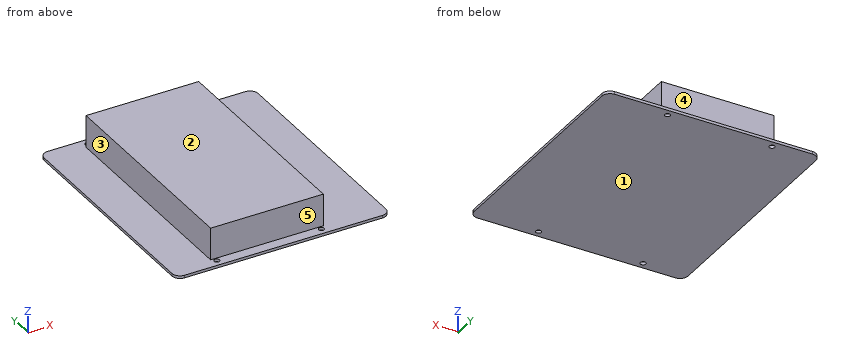
from build123d import *

# Parameters (mm, degrees)
BOSS_EXTRUDE1_DEPTH     = 1.27
SKETCH2_W               = 53.34
SKETCH2_H               = 101.981
BOSS_EXTRUDE2_DEPTH     = 15.24
CUT_EXTRUDE1_DEPTH      = 78.055045652
CUT_EXTRUDE1_DEPTH_BACK = 78.055045652
SKETCH4_R               = 1.27


with BuildPart() as part:
    # Sketch1 → Boss-Extrude1 (new body)
    with BuildSketch(Plane.XY):
        with BuildLine():
            Line((-46.7995, 56.0705), (46.7995, 56.0705))
            ThreePointArc((46.7995, 56.0705), (49.493576836, 54.954576836), (50.6095, 52.2605))
            Line((50.6095, 52.2605), (50.6095, -52.2605))
            ThreePointArc((50.6095, -52.2605), (49.493576836, -54.954576836), (46.7995, -56.0705))
            Line((46.7995, -56.0705), (-46.7995, -56.0705))
            ThreePointArc((-46.7995, -56.0705), (-49.493576836, -54.954576836), (-50.6095, -52.2605))
            Line((-50.6095, -52.2605), (-50.6095, 52.2605))
            ThreePointArc((-50.6095, 52.2605), (-49.493576836, 54.954576836), (-46.7995, 56.0705))
        make_face()
    extrude(amount=BOSS_EXTRUDE1_DEPTH)

    # Sketch2 → Boss-Extrude2 (add)
    with BuildSketch(Plane.XY.offset(1.27)):
        with Locations((-4.8895, 0)):
            Rectangle(SKETCH2_W, SKETCH2_H)
    extrude(amount=BOSS_EXTRUDE2_DEPTH)

    # Sketch4 → Cut-Extrude1 (cut, two sides: drawn at the far end of the back side and taken through both)
    with BuildSketch(Plane.XY.offset(1.27).offset(-CUT_EXTRUDE1_DEPTH_BACK)):
        with Locations((-29.6545, 52.7685)):
            Circle(SKETCH4_R)
        with Locations((19.8755, 52.7685)):
            Circle(SKETCH4_R)
        with Locations((-29.6545, -52.7685)):
            Circle(SKETCH4_R)
        with Locations((19.8755, -52.7685)):
            Circle(SKETCH4_R)
    extrude(amount=CUT_EXTRUDE1_DEPTH + CUT_EXTRUDE1_DEPTH_BACK, mode=Mode.SUBTRACT)


solid = part.part
Design review of the part built by this model. Coordinates are the model's own, in mm. Face numbers are marked on the shaded views. A direction names the side the tool comes from. Give positions to 0.01 mm unless a question says otherwise; leave off trailing zeros. Write each loop counter-clockwise with the first axis right and the second up, starting at its lowest first coordinate (ties: lowest second). Pieces come first, ordered by that corner, then holes. Notation, with made-up numbers: M -22,49.25 L 19,49.25 A30 ccw 19,84.25 Z; hole C 1,-11.5 d9. An arc over 180 degrees is marked long. Return JSON: item names as keys, results as strings. Group by question number.
Item 1: Take a section at D-D (x = 43). Give the boundary of the cut face in (y, z).
Item 2: Tool access review of the marked faces 1, 2, 3, 4 and 5: name each direction out of +Z, -Z, +X, -X, +Y, -Y from which nothing blocks a thin tool from reaching the whole face with its end or side.
Item 3: Clearance check with flat-ended pins moving along their axes: pin 1 Ø8 at (y, z) = (37, 12) entering from +X; pin 2 Ø4.5 at (y, z) = (-6, 5) entering from -X; pin 3 Ø7.5 at (x, z) = (-12, 10) entering from -Y; pin 4 Ø3 at (x, z) = (34, 3) entering from +Y. State where each tip first meets the part, or that it passes through.
Item 4: Take a section at B-B (x = 8). Give the boundary of the cut face in (y, z), plus the area to 3 significant figures.
Item 5: Take a section at A-A (y = -20). Give the boundary of the cut face in (x, z), plus the area to 3 significant figures.
Item 6: Wall thickness on line 1 along X through (y, z) = (52, 1); line 2 along Z through (x, y) = (37.5, -39); line 3 along X through (y, z) = (-10.5, 15): over which ranges is each line inside the solid? List them lowest first.
Item 7: Take a section at C-C (z = 5). Give the boundary of the cut face in (x, y).
Return value:
{
 "1": {"outline": "M -56.07,0 L 56.07,0 L 56.07,1.27 L -56.07,1.27 Z"},
 "2": {"face 1": "-Z, +X, -X, +Y, -Y", "face 2": "+Z, +X, -X, +Y, -Y", "face 3": "+Z, -X, +Y, -Y", "face 4": "+Z, +X, -X, +Y", "face 5": "+Z, +X, -X, -Y"},
 "3": {"pin 1": "stops at x = 21.78", "pin 2": "stops at x = -31.56", "pin 3": "stops at y = -50.99", "pin 4": "passes through"},
 "4": {"outline": "M -56.07,0 L 56.07,0 L 56.07,1.27 L 50.99,1.27 L 50.99,16.51 L -50.99,16.51 L -50.99,1.27 L -56.07,1.27 Z", "area": "1,700 mm2"},
 "5": {"outline": "M -50.61,0 L 50.61,0 L 50.61,1.27 L 21.78,1.27 L 21.78,16.51 L -31.56,16.51 L -31.56,1.27 L -50.61,1.27 Z", "area": "941 mm2"},
 "6": {"line 1": "x = -50.61 to -30.67, -28.64 to 18.86, 20.89 to 50.61", "line 2": "z = 0 to 1.27", "line 3": "x = -31.56 to 21.78"},
 "7": {"outline": "M -31.56,-50.99 L 21.78,-50.99 L 21.78,50.99 L -31.56,50.99 Z"}
}
